Check sheet for the modelled part. Datum: model origin and axes. Units: mm. A direction names the side the tool comes from. Give positions to 0.01 mm unless a question says otherwise; leave off trailing zeros. Order: outer loops, then holes, each group sorted by start corner. A loop starts at its lowest first (then second) coordinate and runs counter-clockwise, first axis right, second up.
Autodesk Fusion 360 part; units mm, degrees
sketch "Sketch1" plane through (0, 0, 0) normal (0, 0, 1) x (1, 0, 0)
  line L0 (0, 0) -> (300, 0)
  line L1 (300, 0) -> (300, 1200)
  line L2 (300, 1200) -> (0, 1200)
  line L3 (0, 600) -> (-300, 600)
  line L4 (-300, 600) -> (-300, 1800)
  line L5 (-300, 1800) -> (0, 1800)
  line L6 (0, 1800) -> (0, 1200)
  line L7 (0, 0) -> (0, 600)
  line L8 (20, 1820) -> (20, 1220)
  line L9 (320, 1220) -> (20, 1220)
  line L10 (320, -20) -> (320, 1220)
  line L11 (-20, -20) -> (320, -20)
  line L12 (-20, -20) -> (-20, 580)
  line L13 (-20, 580) -> (-320, 580)
  line L14 (-320, 580) -> (-320, 1820)
  line L15 (-320, 1820) -> (20, 1820)
  dimension "d1" = 300
  dimension "d2" = 1200
  dimension "d3" = 300
  dimension "d4" = 1200
  dimension "d5" = -20
extrude "Extrude1" add sketch "Sketch1" along normal blind 400 makes body 1
extrude "Extrude2" add sketch "Sketch1" against normal blind 5 separate body contours L0 L1 L2 L3 L4 L5 L6 L7 makes body 2
extrude "Extrude3" add sketch "Sketch1" against normal blind 5 bodies 1 2
extrude "Extrude4" cut 1 faces at (-313.3333, 1400, 400) along direction (0, 0, -1) blind 100 on bodies 1 bodies 1
extrude "Extrude5" cut 1 faces at (-313.3333, 1400, 300) along direction (0, 0, -1) blind 50 on bodies 1 bodies 1
1) Depth check by flat-ended pin: pin 1 Ø12 at (x, z) = (203, 90) entering from +Y; pin 2 Ø8 at (x, y) = (249.5, 686) entering from +Z; pin 3 Ø4 at (x, z) = (-34, 142.5) entering from -Y. Enter the tip coordinate at first touch or a pass-through.
Recorded:
pin 1: stops at y = 1220
pin 2: stops at z = 0
pin 3: stops at y = 580
2) Material ranges on L1, parallel to Y at x = 67, z = 43; L2, parallel to X at y = 921.5, z = 182.5; L3, parallel to X at y = 94.5, z = 84.5, recorded low to high.
Recorded:
L1: y = -20 to 0, 1200 to 1220
L2: x = -320 to -300, 300 to 320
L3: x = -20 to 0, 300 to 320
3) Section check A-A, the plane z = 228. Record the cut outline in (x, y).
Recorded:
outline: (-320, 580) - (-20, 580) - (-20, -20) - (320, -20) - (320, 1220) - (20, 1220) - (20, 1820) - (-320, 1820) - close; hole (-300, 600) - (0, 600) - (0, 0) - (300, 0) - (300, 1200) - (0, 1200) - (0, 1800) - (-300, 1800) - close
4) Draft check along X on faces 5 (the face through (-20, 276, 121)), 6 (the face through (300, 592, 123)), 7 (the face through (0, 296, 123)), 8 (the face through (172, 1220, 121)). Enter one of: +X half, -X half, draft (parallel to the pull), parting line (faces both ways), or undercut.
Recorded:
face 5: -X half
face 6: undercut
face 7: undercut
face 8: draft
5) Section check B-B, the plane y = 1496. Record the cut outline in (x, z), then the cut area to 3 significant figures.
Recorded:
outline: (-320, -5) - (20, -5) - (20, 250) - (0, 250) - (0, 0) - (-300, 0) - (-300, 250) - (-320, 250) - close
area: 11,700 mm2
6) Section check C-C, the plane x = 67.5. Record the cut outline in (y, z).
Recorded:
outline: (-20, -5) - (1220, -5) - (1220, 250) - (1200, 250) - (1200, 0) - (0, 0) - (0, 250) - (-20, 250) - close
7) Set-up check for faces 1 (the face through (20, 1524, 121)), 2 (the face through (152, 1200, 123)), 3 (the face through (-168, 580, 121)), 4 (the face through (-4, 913, -5)): record each of +Z, -Z, +X, -X, +Y, -Y from which the full face is reachable in a straight line by a thin tool's end or side.
Recorded:
face 1: +Z, -Z, +X, +Y
face 2: +Z
face 3: +Z, -Z, -X, -Y
face 4: -Z, +X, -X, +Y, -Y
